Part model, mm, in its own coordinate system. Face numbers are marked on the shaded views. A direction names the side the tool comes from. Coordinates: 2 decimals unless noted, no trailing zeros. Loops run counter-clockwise (first coordinate to the right, second up) from the corner with the lowest first, then second, coordinate; pieces in that order, holes last. Notation, with made-up numbers: (7, 69.5) - (62, 69.5) arc R20 cw to (62, 73.5) - close; hole circle Ø2 at (69.25, 43). An arc over 180 degrees is marked (long way). Use a Markdown table: item, result. Add a question column.
1. Band-saw the part on B-B, the plane z = -64.5. Give the cut face in (x, y), plus the area to 3 significant figures.
2. Wall check: probe 1 along X at (y, z) = (84, -40); probe 2 along Z at (x, y) = (-13, 96.5); probe 3 along X at (y, z) = (38.5, -60). Give the ranges that are in metal, low to high. Write a range as [from, to].
3. Drop flat-ended pins along their axis: pin 1 (3.5 mm diameter, centred on x = 108, z = 33, fed in from -Y); pin 2 (12 mm diameter, centred on y = 44.5, z = -20, fed in from +X). Give the stop position or say it passes through.
4. Band-saw the part on D-D, the plane y = 136.5. Give the cut face in (x, z).
5. 3-axis set-ups, long thin cutter, end or side, ignore diameter. For the marked faces 5 and 6: which of +Z, -Z, +X, -X, +Y, -Y reach the whole face in a straight line?
6. Pull direction Z, two halves, no side cores. Call the marked faces 1, 2, 3 and 4: pulls with the +Z half, pulls with the -Z half, needs draft (parallel to the pull), parting line crosses it, or undercut.
7. Band-saw the part on A-A, the plane y = 25. Give the cut face in (x, z).
8. Band-saw the part on C-C, the plane x = 75. Give the cut face in (y, z).
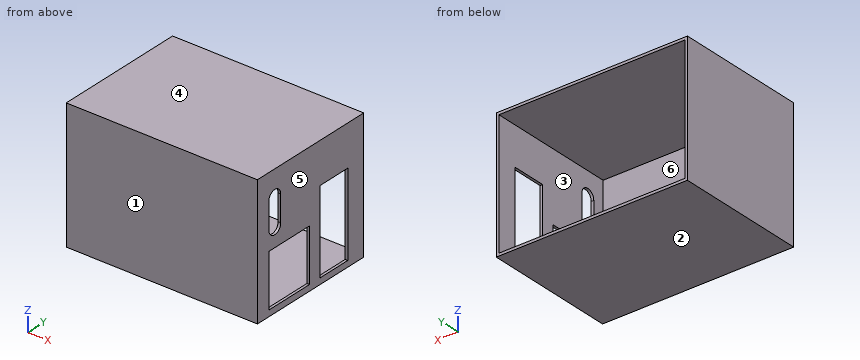
Autodesk Inventor part; units mm, degrees
ref_plane "YZ Plane" through (0, 0, 0) normal (1, 0, 0) x (0, 1, 0)
ref_plane "XZ Plane" through (0, 0, 0) normal (0, 1, 0) x (-1, 0, 0)
ref_plane "XY Plane" through (0, 0, 0) normal (0, 0, 1) x (1, 0, 0)
sketch "Sketch1" plane through (0, 0, 0) normal (0, 1, 0) x (-1, 0, 0)
  line L0 (110, 75) -> (-110, 75)
  line L1 (-110, 75) -> (-110, -75)
  line L2 (-110, -75) -> (110, -75)
  line L3 (110, -75) -> (110, 75)
  line L4 (110, 75) -> (-110, -75) construction
  line L5 (-110, 75) -> (110, -75) construction
  point P0 (0, 0)
  dimension "d0" = 150
  dimension "d1" = 220
extrude "Extrusion1" add sketch "Sketch1" along normal blind 3
sketch "Sketch2" plane through (0, 3, 0) normal (0, 1, 0) x (1, 0, 0)
  line L0 (110, -75) -> (110, 75)
  line L1 (-110, -75) -> (110, -75)
  line L2 (110, -75) -> (110, 75)
  line L3 (110, 75) -> (-110, 75)
  line L4 (-110, 75) -> (-110, -75)
  line L5 (-110, -75) -> (110, 75) construction
  line L6 (110, -75) -> (-110, 75) construction
  line L7 (-107, -72) -> (107, -72)
  line L8 (107, -72) -> (107, 72)
  line L9 (107, 72) -> (-107, 72)
  line L10 (-107, 72) -> (-107, -72)
  line L11 (-107, -72) -> (107, 72) construction
  line L12 (107, -72) -> (-107, 72) construction
  point P0 (0, 0)
  dimension "d4" = 144
  dimension "d5" = 214
extrude "Extrusion2" add sketch "Sketch2" along normal blind 150
sketch "Sketch3" plane through (110, 0, 75) normal (1, 0, 0) x (0, 0, -1)
  line L0 (47, 130) -> (143, 130)
  line L1 (143, 130) -> (143, 90)
  line L2 (143, 90) -> (47, 90)
  line L3 (47, 90) -> (47, 130)
  line L4 (47, 130) -> (143, 90) construction
  line L5 (143, 130) -> (47, 90) construction
  line L6 (0, 0) -> (0, 153)
  line L7 (82, 75) -> (143, 75)
  line L8 (143, 75) -> (143, 17)
  line L9 (143, 17) -> (82, 17)
  line L10 (82, 17) -> (82, 75)
  line L11 (82, 75) -> (143, 17) construction
  line L12 (143, 75) -> (82, 17) construction
  line L13 (30, 25) -> (60, 25) construction
  line L14 (30, 16.456) -> (60, 16.456)
  line L15 (60, 33.544) -> (30, 33.544)
  arc A0 (30, 33.544) -> (30, 16.456) centre (30, 25) ccw
  arc A1 (60, 16.456) -> (60, 33.544) centre (60, 25) ccw
  point P0 (75, 0)
  point P1 (95, 110)
  point P2 (112.5, 46)
  point P3 (0, 3)
  point P4 (45, 25)
  dimension "d8" = 96
  dimension "d9" = 40
  dimension "d10" = 95
  dimension "d11" = 110
  dimension "d14" = 61
  dimension "d15" = 58
  dimension "d16" = 0
  dimension "d17" = 46
  dimension "d18" = 25
  dimension "d19" = 30
  dimension "d20" = 30
  dimension "d21" = 8.544
extrude "Extrusion3" cut sketch "Sketch3" against normal blind 3
properties part number "perspex_shell"
Geometry check:
| question | item | result |
|---|---|---|
| 1 | outline | (-110, 0) - (110, 0) - (110, 17) - (107, 17) - (107, 3) - (-107, 3) - (-107, 153) - (-110, 153) - close; (107, 75) - (110, 75) - (110, 90) - (107, 90) - close; (107, 130) - (110, 130) - (110, 153) - (107, 153) - close |
| 1 | area | 1,270 mm^2 |
| 2 | probe 1 | x = [-110, -107], [107, 110] |
| 2 | probe 2 | z = [-75, -72], [72, 75] |
| 2 | probe 3 | x = [-110, -107] |
| 3 | pin 1 | stops at y = 0 |
| 3 | pin 2 | stops at x = -107 |
| 4 | outline | (-110, -75) - (110, -75) - (110, 75) - (-110, 75) - close; hole (-107, -72) - (107, -72) - (107, 72) - (-107, 72) - close |
| 5 | face 5 | +Z, -Z, +X, +Y, -Y |
| 5 | face 6 | +Y |
| 6 | face 1 | needs draft |
| 6 | face 2 | pulls with the -Z half |
| 6 | face 3 | undercut |
| 6 | face 4 | pulls with the +Z half |
| 7 | outline | (-110, -75) - (110, -75) - (110, -68) - (107, -68) - (107, -72) - (-107, -72) - (-107, 72) - (107, 72) - (107, 53.54) - (110, 53.54) - (110, 75) - (-110, 75) - close; (107, -7) - (110, -7) - (110, 6.46) - (107, 6.46) - close |
| 8 | outline | (0, -75) - (153, -75) - (153, -72) - (3, -72) - (3, 72) - (153, 72) - (153, 75) - (0, 75) - close |
